Could you check a few things on this model? Use its own coordinates, in mm. Give positions to 0.01 mm unless a question says otherwise; leave off trailing zeros. Loops run counter-clockwise (first coordinate to the right, second up) from the corner with the lowest first, then second, coordinate; pieces in that order, holes last. Notation, with made-up numbers: (68.25, -5) - (111.25, -5) arc R23 ccw to (111.25, 4) - close; hole circle Ø1 at (80, 88). An arc over 180 degrees is marked (long way). One line per item, written item: value. Start each with the question number.
Q1. I want a section at C-C (z = -107). Please give me the cut outline in (x, y) (3 decimals), then the cut area to 3 significant figures.
Q2. I want a section at A-A (y = 1). Count the separate pieces of the cut face and the enclosed holes in it, then the cut area to 3 significant figures.
Q3. I want a section at B-B (z = -52.5). Please give me the cut outline in (x, y) (3 decimals), then the cut area to 3 significant figures.
Q4. If I drill on line 1 (X direction, y = 0.9, z = -31.75); line 2 (X direction, y = 2.2, z = -298.45); line 3 (X direction, y = 1.7, z = -145), over which ranges is the centre line in solid material (lowest first)? Write a range as from..to.
Q5. I'm going to push flat-ended pins straight in: P1, Ø1.5, axis at y = 2, z = -277.5, coming from the +X side; P2, Ø1.5, axis at y = 1, z = -290, coming from the +X side. Where does each tip first touch, or does it pass through?
```python
from build123d import *

# Parameters (mm, degrees)
BOSS_EXTRUDE1_DEPTH          = 3.175
FILLET1_R                    = 12.7
F_1_8_0_125_DIAMETER_HOLE1_D = 3.175


with BuildPart() as part:
    # Sketch1 → Boss-Extrude1 (new body)
    with BuildSketch(Plane(origin=(0, 0, 0), x_dir=(1, 0, 0), z_dir=(0, 1, 0))):
        Polygon((31.75, 0), (82.55, 0), (82.55, 31.75), (31.75, 330.2), (0, 330.2), (0, 0), align=None)
    extrude(amount=BOSS_EXTRUDE1_DEPTH)

    # Fillet1
    fillet1_edges = [part.edges().sort_by_distance(p)[0] for p in [
        (0, 1.5875, -330.2),
        (31.75, 1.5875, -330.2),
        (82.55, 1.5875, -31.75),
        (82.55, 1.5875, 0),
        (0, 1.5875, 0),
    ]]
    fillet(fillet1_edges, radius=FILLET1_R)

    # 1/8 (0.125) Diameter Hole1 (through all)
    with Locations(Plane(origin=(0, 0, 0), x_dir=(-1, 0, 0), z_dir=(0, -1, 0))):
        with Locations((-8.4328, 298.45), (-8.4328, 209.55), (-8.4328, 120.65), (-8.4328, 31.75), (-66.675, 12.7), (-15.875, 12.7)):
            Hole(F_1_8_0_125_DIAMETER_HOLE1_D / 2)


solid = part.part
```
Worked answers:
1. outline: (0, 0) - (69.741, 0) - (69.741, 3.175) - (0, 3.175) - close
1. area: 221 mm²
2. separate pieces: 1
2. enclosed holes: 6
2. area: 19,500 mm²
3. outline: (0, 0) - (79.018, 0) - (79.018, 3.175) - (0, 3.175) - close
3. area: 251 mm²
4. line 1: x = 0..6.85, 10.02..82.5
4. line 2: x = 0..6.85, 10.02..37.15
4. line 3: x = 0..63.27
5. P1: stops at x = 40.85
5. P2: stops at x = 38.72
